Input: part model. Units: mm. Frame: model coordinates. Give positions to 0.01 mm unless a question says otherwise; leave off trailing zeros. Loops run counter-clockwise (first coordinate to the right, second up) from the corner with the lowest first, then second, coordinate; pieces in that order, holes last. Notation, with made-up numbers: (-38, 78.5) -> (7, 78.5) arc R15 cw to (7, 92.5) -> close; hole circle Ø6 at (12, 54.5). An arc over 180 degrees is marked (long way). Use CSV: the item, a comma, the result in double quotes.
```python
from build123d import *

# Parameters (mm, degrees)
ESQUISSE1_R             = 3.5
ESQUISSE1_R_2           = 2.5
BASE_EXTRU_MINCE_DEPTH  = 2.5
CHANFREIN1_SIZE         = 0.2
ESQUISSE2_R             = 0.75
ENL_V_MAT_EXTRU_1_DEPTH = 5


with BuildPart() as part:
    # Esquisse1 → Base-Extru.-Mince (new, symmetric)
    with BuildSketch(Plane.XY):
        Circle(ESQUISSE1_R)
        Circle(ESQUISSE1_R_2, mode=Mode.SUBTRACT)
    extrude(amount=BASE_EXTRU_MINCE_DEPTH, both=True)

    # Chanfrein1
    chanfrein1_edges = [part.edges().sort_by_distance(p)[0] for p in [
        (-3.5, 0, -2.5),
        (-3.5, 0, 2.5),
    ]]
    chamfer(chanfrein1_edges, length=CHANFREIN1_SIZE)

    # Esquisse2 → Enlèv. mat.-Extru.1 (cut, symmetric)
    with BuildSketch(Plane(origin=(0, 0, 0), x_dir=(1, 0, 0), z_dir=(0, 1, 0))):
        with Locations(Location((0, 0, 0), (0, 0, 270))):
            Circle(ESQUISSE2_R)
    extrude(amount=ENL_V_MAT_EXTRU_1_DEPTH, both=True, mode=Mode.SUBTRACT)


solid = part.part
```
1) Section query A-A (x = 0). Return loops of the section in (y, z).
From the geometry:
outline,"(-3.5, -2.3) -> (-3.3, -2.5) -> (-2.5, -2.5) -> (-2.5, -0.75) -> (-3.5, -0.75) -> close; (-3.5, 0.75) -> (-2.5, 0.75) -> (-2.5, 2.5) -> (-3.3, 2.5) -> (-3.5, 2.3) -> close; (2.5, -2.5) -> (3.3, -2.5) -> (3.5, -2.3) -> (3.5, -0.75) -> (2.5, -0.75) -> close; (2.5, 0.75) -> (3.5, 0.75) -> (3.5, 2.3) -> (3.3, 2.5) -> (2.5, 2.5) -> close"
2) Section query B-B (y = 0). Return loops of the section in (x, z).
From the geometry:
outline,"(-3.5, -2.3) -> (-3.3, -2.5) -> (-2.5, -2.5) -> (-2.5, 2.5) -> (-3.3, 2.5) -> (-3.5, 2.3) -> close; (2.5, -2.5) -> (3.3, -2.5) -> (3.5, -2.3) -> (3.5, 2.3) -> (3.3, 2.5) -> (2.5, 2.5) -> close"
3) Section query D-D (z = 1.55). Return loops of the section in (x, y).
From the geometry:
outline,"circle Ø7 at (0, 0); hole circle Ø5 at (0, 0)"
4) Ray query, line 1 (Y direction, x = 0, z = 0.8); line 2 (Z direction, x = 0, y = -2.9); line 3 (X direction, y = -2.5, z = -0.1). Return the intervals inside material, ascending.
From the geometry:
line 1,"y = -3.5 to -2.5, 2.5 to 3.5"
line 2,"z = -2.5 to -0.75, 0.75 to 2.5"
line 3,"x = -2.45 to -0.74, 0.74 to 2.45"
5) Mould query, pull axis X, two halves, no side actions, for faces 1 (the cylindrical face through (0.51, 2.95, -0.55)), 2 (the cylindrical face through (1.615, -3.105, 0.032)), 3 (the cylindrical face through (0.225, -2.935, 0.715)), 4 (the flat face through (-2, 2, -2.5)). Classes: pulls with the +X half, pulls with the -X half, needs draft (parallel to the pull), parting line crosses it, or undercut.
From the geometry:
face 1,"undercut"
face 2,"parting line crosses it"
face 3,"undercut"
face 4,"needs draft"
6) Section query C-C (z = 0). Return loops of the section in (x, y), then the cut area to 3 significant figures.
From the geometry:
outline,"(-0.75, -3.42) -> (-0.75, -2.38) arc R2.5 cw to (-0.75, 2.38) -> (-0.75, 3.42) arc R3.5 ccw to start; (0.75, -3.42) arc R3.5 ccw to (0.75, 3.42) -> (0.75, 2.38) arc R2.5 cw to (0.75, -2.38) -> close"
area,"15.8 mm^2"
